Can you work these out from the drawing? Everything is in mm from the part's minimum corner. A direction names the side the tool comes from. Round coordinates to 2 decimals unless told otherwise and drop trailing zeros. Write each loop counter-clockwise with the first axis right and the second up, starting at its lowest first coordinate (ties: lowest second). Pieces come first, ordered by that corner, then holes. Notation, with made-up numbers: (87.25, 54) -> (114.25, 54) arc R8 cw to (114.25, 61) -> close; hole circle Ø10 at (-14.75, 67.5). An arc over 180 degrees is marked (long way). Answer as CSV lines item,"result". Start each with the question number.
Q1. For the marked faces 1 and 2, which set-ups out of +Z, -Z, +X, -X, +Y, -Y let a thin tool reach every point of the face, with its end or its side?
Q2. If we mould it in two halves opening along X, with no side actions, what happens to the marked faces 3, 4 and 5? For each: pulls with the +X half, pulls with the -X half, needs draft (parallel to the pull), parting line crosses it, or undercut.
Q3. Imagine slicing it at C-C on x = 103. Please give me the cut outline in (y, z).
Q4. Imagine slicing it at A-A on x = 9. Please give me the cut outline in (y, z).
Q5. If I drill on line 1 (Z direction, x = 141, y = 19); line 2 (Z direction, x = 86.5, y = 77), over which ranges is the centre line in solid material (lowest first)? Write a range as [from, to].
Q6. Imagine slicing it at B-B on z = 9. Please give me the cut outline in (x, y).
Q7. Will these pins go through, and if not, where does the flat tip stop? pin 1 Ø5 at (x, z) = (120, 65.5) entering from +Y; pin 2 Ø11 at (x, z) = (11, 10.5) entering from +Y.
Q8. Imagine slicing it at D-D on z = 42. Please give me the cut outline in (x, y).
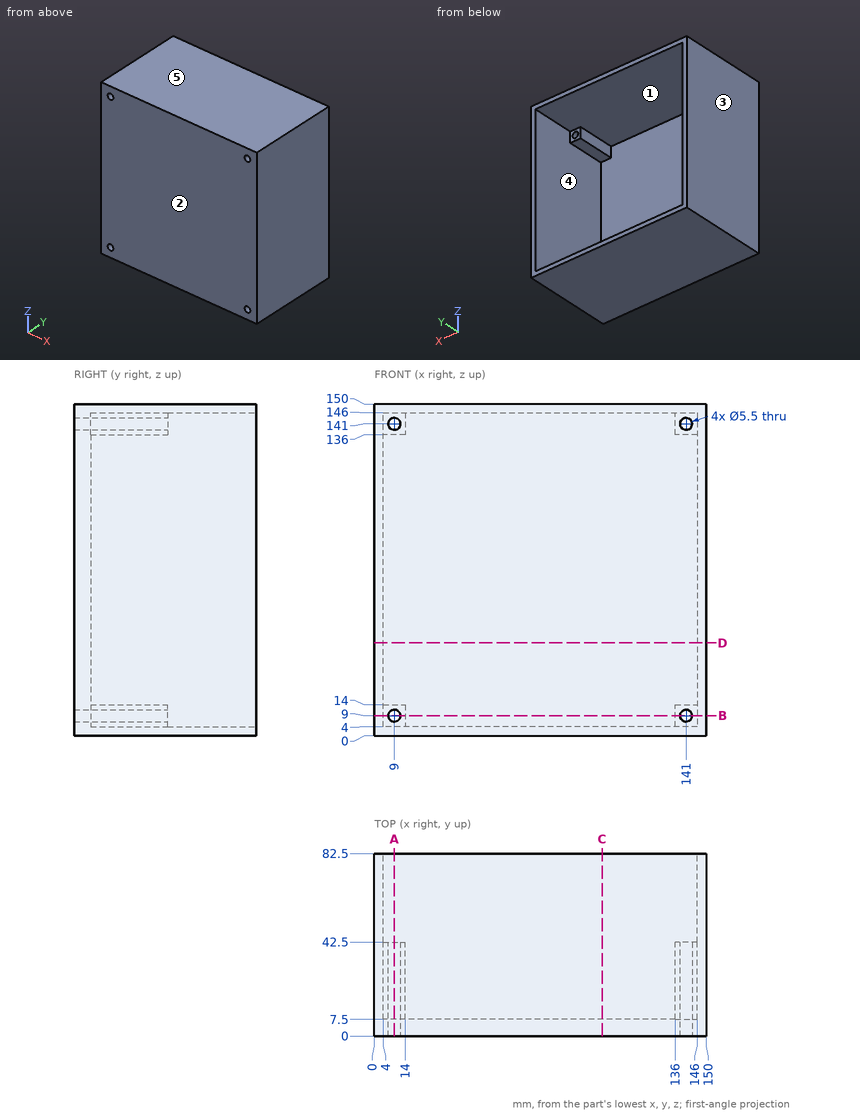
Checks:
1,face 1,"+Y"
1,face 2,"+Z, -Z, +X, -X, -Y"
2,face 3,"pulls with the -X half"
2,face 4,"undercut"
2,face 5,"needs draft"
3,outline,"(0, 0) -> (82.5, 0) -> (82.5, 4) -> (7.5, 4) -> (7.5, 146) -> (82.5, 146) -> (82.5, 150) -> (0, 150) -> close"
4,outline,"(0, 0) -> (82.5, 0) -> (82.5, 4) -> (42.5, 4) -> (42.5, 6.25) -> (0, 6.25) -> close; (0, 11.75) -> (42.5, 11.75) -> (42.5, 14) -> (7.5, 14) -> (7.5, 136) -> (42.5, 136) -> (42.5, 138.25) -> (0, 138.25) -> close; (0, 143.75) -> (42.5, 143.75) -> (42.5, 146) -> (82.5, 146) -> (82.5, 150) -> (0, 150) -> close"
5,line 1,"[0, 6.25], [11.75, 14], [136, 138.25], [143.75, 150]"
5,line 2,"[0, 4], [146, 150]"
6,outline,"(0, 0) -> (6.25, 0) -> (6.25, 42.5) -> (4, 42.5) -> (4, 82.5) -> (0, 82.5) -> close; (11.75, 0) -> (138.25, 0) -> (138.25, 42.5) -> (136, 42.5) -> (136, 7.5) -> (14, 7.5) -> (14, 42.5) -> (11.75, 42.5) -> close; (143.75, 0) -> (150, 0) -> (150, 82.5) -> (146, 82.5) -> (146, 42.5) -> (143.75, 42.5) -> close"
7,pin 1,"y = 7.5"
7,pin 2,"y = 42.5"
8,outline,"(0, 0) -> (150, 0) -> (150, 82.5) -> (146, 82.5) -> (146, 7.5) -> (4, 7.5) -> (4, 82.5) -> (0, 82.5) -> close"
